Check sheet for the modelled part. Datum: model origin and axes. Units: mm. Give positions to 0.01 mm unless a question says otherwise; leave off trailing zeros. Loops run counter-clockwise (first coordinate to the right, second up) from the corner with the lowest first, then second, coordinate; pieces in that order, holes last. Notation, with made-up numbers: (22, 28.5) -> (72, 28.5) arc R14 cw to (72, 50.5) -> close; hole circle Ø9 at (23, 31.25). An arc over 180 degrees is marked (long way). Answer as CSV lines item,"result". Start each with the question number.
(1) Section check B-B on z = -5. Enter the section's corners in (x, y), plus the area to 3 significant figures.
(2) Section check C-C on y = 1.65. State how many separate pieces and enclosed holes the cut face has, plus the area to 3 significant figures.
(3) Section check A-A on x = -17. Enter the section's corners in (y, z), plus the area to 3 significant figures.
(4) Section check D-D on x = -60. Enter the section's corners in (y, z), plus the area to 3 significant figures.
(5) Gauge pin test, flat ends, axial feed: pin 1 Ø4.5 at (x, z) = (-60, 13) entering from -Y; pin 2 Ø3.5 at (x, z) = (47.5, 12.5) entering from +Y. Record the tip position at first contact, or that the pin passes through.
(6) Material ranges on line 1 (Z direction, x = -18, y = 2.4); line 2 (X direction, y = 0.75, z = 3.5); line 3 (X direction, y = 1.4, z = -13.5), recorded low to high. Write a range as from..to.
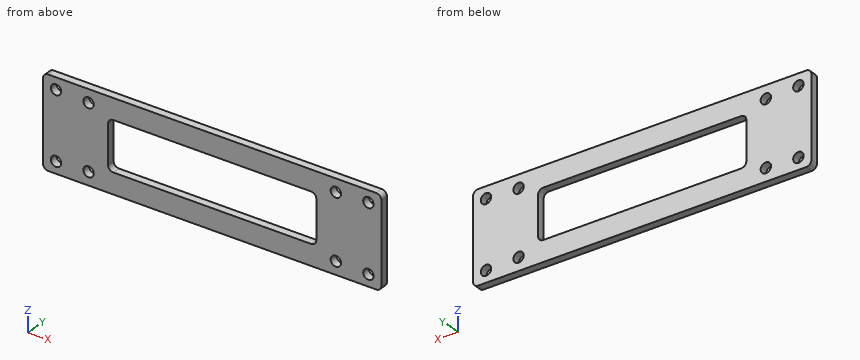
from build123d import *

# Parameters (mm, degrees)
SKETCH_1_W          = 110
SKETCH_1_H          = 35
SKETCH_1_R          = 2
EXTRUDE_1_DEPTH     = 3
SKETCH_2_W          = 10
SKETCH_2_H          = 35
SKETCH_2_R          = 2
EXTRUDE_2_DEPTH     = 3
SKETCH_3_W          = 80
SKETCH_3_H          = 19
CUT_EXTRUDE_1_DEPTH = 3
FILLET_1_R          = 2


with BuildPart() as part:
    # 草图1 → 凸台-拉伸1 (new body)
    with BuildSketch(Plane(origin=(0, 0, 0), x_dir=(1, 0, 0), z_dir=(0, 1, 0))):
        Rectangle(SKETCH_1_W, SKETCH_1_H)
        with Locations(Location((-47.5, 12.5, 0), (0, 0, 270))):
            Circle(SKETCH_1_R, mode=Mode.SUBTRACT)
        with Locations(Location((-47.5, -12.5, 0), (0, 0, 270))):
            Circle(SKETCH_1_R, mode=Mode.SUBTRACT)
        with Locations(Location((47.5, -12.5, 0), (0, 0, 90))):
            Circle(SKETCH_1_R, mode=Mode.SUBTRACT)
        with Locations(Location((47.5, 12.5, 0), (0, 0, 90))):
            Circle(SKETCH_1_R, mode=Mode.SUBTRACT)
    extrude(amount=EXTRUDE_1_DEPTH)

    # 草图2 → 凸台-拉伸2 (add)
    # profile 1 of 2: a face of its own
    with BuildSketch(Plane(origin=(0, 3, 0), x_dir=(1, 0, 0), z_dir=(0, 1, 0))):
        with Locations((60, 0)):
            Rectangle(SKETCH_2_W, SKETCH_2_H)
        with Locations(Location((60, 13, 0), (0, 0, 270))):
            Circle(SKETCH_2_R, mode=Mode.SUBTRACT)
        with Locations(Location((60, -13, 0), (0, 0, 270))):
            Circle(SKETCH_2_R, mode=Mode.SUBTRACT)
    # profile 2 of 2: a face of its own
    with BuildSketch(Plane(origin=(0, 3, 0), x_dir=(1, 0, 0), z_dir=(0, 1, 0))):
        with Locations((-60, 0)):
            Rectangle(SKETCH_2_W, SKETCH_2_H)
        with Locations(Location((-60, 13, 0), (0, 0, 270))):
            Circle(SKETCH_2_R, mode=Mode.SUBTRACT)
        with Locations(Location((-60, -13, 0), (0, 0, 270))):
            Circle(SKETCH_2_R, mode=Mode.SUBTRACT)
    extrude(amount=-EXTRUDE_2_DEPTH)

    # 草图3 → 切除-拉伸1 (cut)
    with BuildSketch(Plane(origin=(0, 3, 0), x_dir=(1, 0, 0), z_dir=(0, 1, 0))):
        Rectangle(SKETCH_3_W, SKETCH_3_H)
    extrude(amount=-CUT_EXTRUDE_1_DEPTH, mode=Mode.SUBTRACT)

    # 圆角1
    fillet_1_edges = [part.edges().sort_by_distance(p)[0] for p in [
        (-65, 1.5, -17.5),
        (-65, 1.5, 17.5),
        (65, 1.5, -17.5),
        (65, 1.5, 17.5),
        (40, 1.5, -9.5),
        (40, 1.5, 9.5),
        (-40, 1.5, 9.5),
        (-40, 1.5, -9.5),
    ]]
    fillet(fillet_1_edges, radius=FILLET_1_R)


solid = part.part
Working result:
1,outline,"(-65, 0) -> (-40, 0) -> (-40, 3) -> (-65, 3) -> close; (40, 0) -> (65, 0) -> (65, 3) -> (40, 3) -> close"
1,area,"150 mm^2"
2,separate pieces,"1"
2,enclosed holes,"9"
2,area,"2,930 mm^2"
3,outline,"(0, -17.5) -> (3, -17.5) -> (3, -9.5) -> (0, -9.5) -> close; (0, 9.5) -> (3, 9.5) -> (3, 17.5) -> (0, 17.5) -> close"
3,area,"48.0 mm^2"
4,outline,"(0, -17.5) -> (3, -17.5) -> (3, -15) -> (0, -15) -> close; (0, -11) -> (3, -11) -> (3, 11) -> (0, 11) -> close; (0, 15) -> (3, 15) -> (3, 17.5) -> (0, 17.5) -> close"
4,area,"81.0 mm^2"
5,pin 1,"stops at y = 0"
5,pin 2,"passes through"
6,line 1,"z = -17.5..-9.5, 9.5..17.5"
6,line 2,"x = -65..-40, 40..65"
6,line 3,"x = -65..-61.94, -58.06..-49.23, -45.77..45.77, 49.23..58.06, 61.94..65"
